The figure shows three views and two pictorial views of one solid part (mm, origin at its lowest corner). Answer the questions. Coordinates: 2 decimals unless noted, no trailing zeros. Loops run counter-clockwise (first coordinate to the right, second up) from the corner with the lowest first, then second, coordinate; pieces in that order, holes last. Notation, with made-up numbers: M 35,54 L 89,54 A31 cw 89,93 Z; hole C 58,54.5 d4. An arc over 180 degrees is marked long. Return JSON: item names as keys, results as strings. Group by question number.
1. Section A-A (z = 171.45) is taken. Write down the section's boundary in (x, y).
2. Given P1, Ø15.5, axis at x = 115.062, z = 31.75, coming from the +Y side; P2, Ø7.5, axis at x = 216.662, z = 31.75, coming from the -Y side, each flat-ended and moving along its own axis, determine where each tip first touches the part or whether it passes through.
3. Straight lines are drawn through the part: L1, parallel to X at y = 1.3, z = 171.45; L2, parallel to X at y = 0.6, z = 31 (1 decimal); L3, parallel to Z at x = 240.5, y = 1.5. For each, find the intervals that lie inside material, in ascending order. Write a range as from..to.
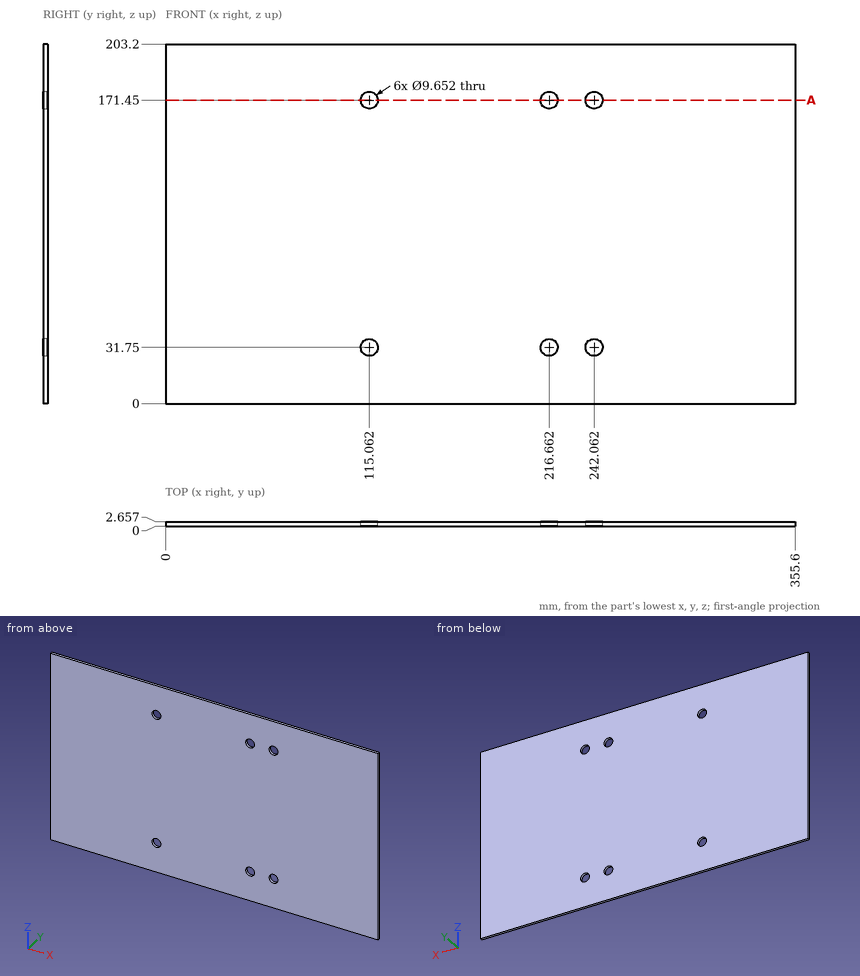
Worked out:
{
 "1": {"outline": "M 0,0 L 110.24,0 L 110.24,2.66 L 0,2.66 Z; M 119.89,0 L 211.84,0 L 211.84,2.66 L 119.89,2.66 Z; M 221.49,0 L 237.24,0 L 237.24,2.66 L 221.49,2.66 Z; M 246.89,0 L 355.6,0 L 355.6,2.66 L 246.89,2.66 Z"},
 "2": {"P1": "y = 2.66", "P2": "through"},
 "3": {"L1": "0..110.24, 119.89..211.84, 221.49..237.24, 246.89..355.6", "L2": "0..110.3, 119.8..211.9, 221.4..237.3, 246.8..355.6", "L3": "0..27.18, 36.32..166.88, 176.02..203.2"}
}
